```python
from build123d import *

# Parameters (mm, degrees)
BOSS_EXTRUDE1_DEPTH = 3.175
SKETCH2_R           = 3.175
CUT_EXTRUDE1_DEPTH  = 6.35
SKETCH3_R           = 2.159
CUT_EXTRUDE2_DEPTH  = 6.35
SKETCH4_R           = 2.2225
CUT_EXTRUDE3_DEPTH  = 351.937720963
SKETCH5_R           = 2.032
CUT_EXTRUDE5_DEPTH  = 351.937720963


with BuildPart() as part:
    # Sketch1 → Boss-Extrude1 (new body)
    with BuildSketch(Plane(origin=(0, 0, 0), x_dir=(1, 0, 0), z_dir=(0, 1, 0))):
        Polygon((-16.864769233, 51.656360067), (-61.766049839, 6.755079462), (-61.766049839, -208.242359328), (-16.864769233, -253.143639933), (198.132669556, -253.143639933), (243.033950161, -208.242359328), (243.033950161, 6.755079462), (198.132669556, 51.656360067), align=None)
        with BuildLine():
            ThreePointArc((43.337601054, -119.793639933), (49.687601054, -126.143639933), (43.337601054, -132.493639933))
            Line((43.337601054, -132.493639933), (-13.679235779, -132.493639933))
            ThreePointArc((-13.679235779, -132.493639933), (-20.029235779, -126.143639933), (-13.679235779, -119.793639933))
            Line((-13.679235779, -119.793639933), (43.337601054, -119.793639933))
        make_face(mode=Mode.SUBTRACT)
        with BuildLine():
            Line((194.947136102, -132.493639933), (137.930299269, -132.493639933))
            ThreePointArc((137.930299269, -132.493639933), (131.580299269, -126.143639933), (137.930299269, -119.793639933))
            Line((137.930299269, -119.793639933), (194.947136102, -119.793639933))
            ThreePointArc((194.947136102, -119.793639933), (201.297136102, -126.143639933), (194.947136102, -132.493639933))
        make_face(mode=Mode.SUBTRACT)
        with BuildLine():
            Line((-13.679235779, -68.993639933), (43.337601054, -68.993639933))
            ThreePointArc((43.337601054, -68.993639933), (49.687601054, -75.343639933), (43.337601054, -81.693639933))
            Line((43.337601054, -81.693639933), (-13.679235779, -81.693639933))
            ThreePointArc((-13.679235779, -81.693639933), (-20.029235779, -75.343639933), (-13.679235779, -68.993639933))
        make_face(mode=Mode.SUBTRACT)
        with BuildLine():
            ThreePointArc((137.930299269, -81.693639933), (131.580299269, -75.343639933), (137.930299269, -68.993639933))
            Line((137.930299269, -68.993639933), (194.947136102, -68.993639933))
            ThreePointArc((194.947136102, -68.993639933), (201.297136102, -75.343639933), (194.947136102, -81.693639933))
            Line((194.947136102, -81.693639933), (137.930299269, -81.693639933))
        make_face(mode=Mode.SUBTRACT)
    extrude(amount=BOSS_EXTRUDE1_DEPTH)

    # Sketch2 → Cut-Extrude1 (cut)
    with BuildSketch(Plane(origin=(0, 3.175, 0), x_dir=(1, 0, 0), z_dir=(0, 1, 0))):
        with Locations(Location((-15.627316695, 32.458395287, 0), (0, 0, 270))):
            Circle(SKETCH2_R)
        with Locations(Location((2.333195547, 14.497883045, 0), (0, 0, 270))):
            Circle(SKETCH2_R)
        with Locations(Location((-24.607572816, -12.442885319, 0), (0, 0, 270))):
            Circle(SKETCH2_R)
        with Locations(Location((-42.568085059, 5.517626924, 0), (0, 0, 270))):
            Circle(SKETCH2_R)
        with Locations(Location((205.875473139, -12.442885319, 0), (0, 0, 270))):
            Circle(SKETCH2_R)
        with Locations(Location((223.835985381, 5.517626924, 0), (0, 0, 270))):
            Circle(SKETCH2_R)
        with Locations(Location((178.934704776, 14.497883045, 0), (0, 0, 270))):
            Circle(SKETCH2_R)
        with Locations(Location((196.895217018, 32.458395287, 0), (0, 0, 270))):
            Circle(SKETCH2_R)
        with Locations(Location((-24.607572816, -189.044394548, 0), (0, 0, 270))):
            Circle(SKETCH2_R)
        with Locations(Location((-42.568085059, -207.00490679, 0), (0, 0, 270))):
            Circle(SKETCH2_R)
        with Locations(Location((-15.627316695, -233.945675153, 0), (0, 0, 270))):
            Circle(SKETCH2_R)
        with Locations(Location((2.333195547, -215.985162911, 0), (0, 0, 270))):
            Circle(SKETCH2_R)
        with Locations(Location((223.835985381, -207.00490679, 0), (0, 0, 270))):
            Circle(SKETCH2_R)
        with Locations(Location((196.895217018, -233.945675153, 0), (0, 0, 270))):
            Circle(SKETCH2_R)
        with Locations(Location((178.934704776, -215.985162911, 0), (0, 0, 270))):
            Circle(SKETCH2_R)
        with Locations(Location((205.875473139, -189.044394548, 0), (0, 0, 270))):
            Circle(SKETCH2_R)
    extrude(amount=-CUT_EXTRUDE1_DEPTH, mode=Mode.SUBTRACT)

    # Sketch3 → Cut-Extrude2 (cut)
    with BuildSketch(Plane(origin=(0, 3.175, 0), x_dir=(1, 0, 0), z_dir=(0, 1, 0))):
        with Locations(Location((65.233950161, -62.643639933, 0), (0, 0, 270))):
            Circle(SKETCH3_R)
        with Locations(Location((116.033950161, -62.643639933, 0), (0, 0, 270))):
            Circle(SKETCH3_R)
        with Locations(Location((65.233950161, -138.843639933, 0), (0, 0, 270))):
            Circle(SKETCH3_R)
        with Locations(Location((116.033950161, -138.843639933, 0), (0, 0, 270))):
            Circle(SKETCH3_R)
    extrude(amount=-CUT_EXTRUDE2_DEPTH, mode=Mode.SUBTRACT)

    # Sketch4 → Cut-Extrude3 (cut, through all)
    with BuildSketch(Plane(origin=(0, 3.175, 0), x_dir=(1, 0, 0), z_dir=(0, 1, 0))):
        with Locations(Location((58.883950161, 26.256360067, 0), (0, 0, 270))):
            Circle(SKETCH4_R)
        with Locations(Location((122.383950161, 26.256360067, 0), (0, 0, 270))):
            Circle(SKETCH4_R)
        with Locations(Location((58.883950161, -11.843639933, 0), (0, 0, 270))):
            Circle(SKETCH4_R)
        with Locations(Location((122.383950161, -11.843639933, 0), (0, 0, 270))):
            Circle(SKETCH4_R)
        with Locations(Location((122.383950161, -189.643639933, 0), (0, 0, 90))):
            Circle(SKETCH4_R)
        with Locations(Location((58.883950161, -189.643639933, 0), (0, 0, 90))):
            Circle(SKETCH4_R)
        with Locations(Location((122.383950161, -227.743639933, 0), (0, 0, 90))):
            Circle(SKETCH4_R)
        with Locations(Location((58.883950161, -227.743639933, 0), (0, 0, 90))):
            Circle(SKETCH4_R)
    extrude(amount=-CUT_EXTRUDE3_DEPTH, mode=Mode.SUBTRACT)

    # Sketch5 → Cut-Extrude5 (cut, through all)
    with BuildSketch(Plane(origin=(0, 0, 0), x_dir=(1, 0, 0), z_dir=(0, 1, 0))):
        with Locations(Location((147.669482851, -32.676069571, 0), (0, 0, 270))):
            Circle(SKETCH5_R)
        with Locations(Location((175.101482851, -32.676069571, 0), (0, 0, 270))):
            Circle(SKETCH5_R)
        with Locations(Location((175.101482851, -61.632069571, 0), (0, 0, 270))):
            Circle(SKETCH5_R)
        with Locations(Location((147.669482851, -61.632069571, 0), (0, 0, 270))):
            Circle(SKETCH5_R)
    extrude(amount=CUT_EXTRUDE5_DEPTH, mode=Mode.SUBTRACT)


solid = part.part
```
Check sheet for the modelled part. Datum: model origin and axes. Units: mm. Coordinates: 2 decimals unless noted, no trailing zeros. Loops run counter-clockwise (first coordinate to the right, second up) from the corner with the lowest first, then second, coordinate; pieces in that order, holes last. Notation, with made-up numbers: M 40,-23.5 L 49,-23.5 A20 ccw 49,6.5 Z; hole C 61.5,-37 d6. An arc over 180 degrees is marked long. Answer as a JSON object with one key per item and string values.
1. Scan lines: L1, parallel to Z at x = 141, y = 2.5; L2, parallel to X at y = 1.15, z = -31; L3, parallel to X at y = 0.5, z = 188. Record each from-to range of solid material in increasing order. Write a range as from..to.
Outcome:
{"L1": "-51.66..68.99, 81.69..119.79, 132.49..253.14", "L2": "-37.52..-18.45, -12.81..194.07, 199.72..218.79", "L3": "-61.77..-27.61, -21.61..57.39, 60.38..120.89, 123.88..202.88, 208.87..243.03"}
2. Sectioned sample at B-B on y = 1.95. Count the separate pieces of the cut face and the enclosed holes in it, and give its area (3 significant figures).
Outcome:
{"separate pieces": "1", "enclosed holes": "36", "area": "84,700 mm²"}
3. Sectioned sample at A-A on x = -31.5. Record the cut outline in (y, z) (3 decimals).
Outcome:
{"outline": "M 0,-37.021 L 3.175,-37.021 L 3.175,238.508 L 0,238.508 Z"}
